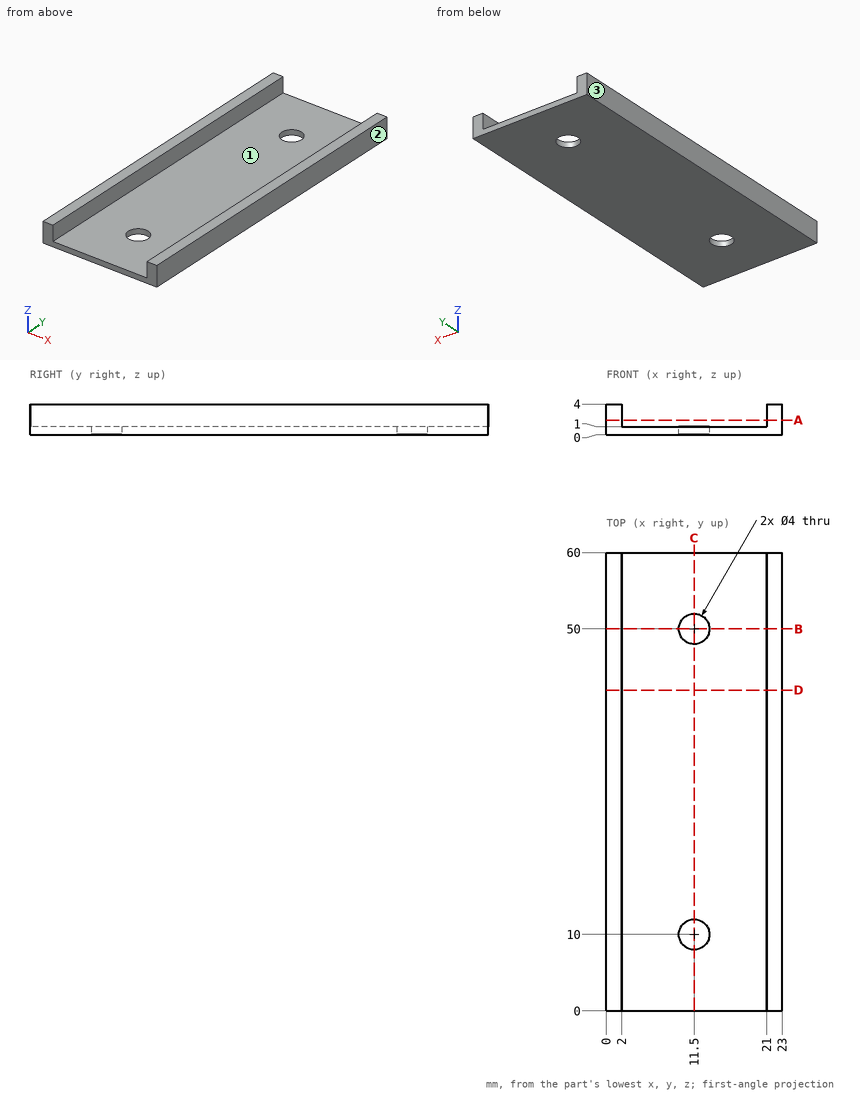
Design review of the part shown in the three views and the two pictorial views. Dimensions are in mm from the part's minimum x, y and z. Give positions to 0.01 mm unless a question says otherwise; leave off trailing zeros. Loops run counter-clockwise (first coordinate to the right, second up) from the corner with the lowest first, then second, coordinate; pieces in that order, holes last. Notation, with made-up numbers: M 9.25,17.5 L 48.25,17.5 A22 cw 48.25,26.5 Z; hole C 40,33.25 d7. An arc over 180 degrees is marked long. Write item = value, one per line.
Q1. We need section B-B (y = 50). Give the boundary of the cut face in (x, z), plus the area to 3 significant figures.
Output values:
outline = M 0,0 L 9.5,0 L 9.5,1 L 2,1 L 2,4 L 0,4 Z; M 13.5,0 L 23,0 L 23,4 L 21,4 L 21,1 L 13.5,1 Z
area = 31.0 mm^2
Q2. Draft analysis for pull direction X (two halves, no side actions). For the marked faces 1, 2 and 3, state which applies: +X half, -X half, draft (parallel to the pull), parting line (faces both ways), or undercut.
Output values:
face_1 = undercut
face_2 = +X half
face_3 = -X half
Q3. We need section C-C (x = 11.5). Give the boundary of the cut face in (y, z), plus the area to 3 significant figures.
Output values:
outline = M 0,0 L 8,0 L 8,1 L 0,1 Z; M 12,0 L 48,0 L 48,1 L 12,1 Z; M 52,0 L 60,0 L 60,1 L 52,1 Z
area = 52.0 mm^2
Q4. To check wall thickness, follow line 1 (Y direction, x = 11.5, z = 0.4); line 2 (X direction, y = 55, z = 2.1); line 3 (Z direction, x = 9.5, y = 4). State the ranges of each line that lie inside material, in increasing order. Write a range as [from, to].
Output values:
line_1 = [0, 8], [12, 48], [52, 60]
line_2 = [0, 2], [21, 23]
line_3 = [0, 1]
Q5. Insertion check: pin 1 (1 mm diameter, centred on x = 17.5, z = 3, fed in from -Y); pin 2 (6 mm diameter, centred on x = 9, y = 45, fed in from +Z). Each pin has a flat end and moves straight along its axis. Give the tip position at first contact, or say it passes through.
Output values:
pin_1 = through
pin_2 = 1
Q6. We need section A-A (z = 1.9). Give the boundary of the cut face in (x, y).
Output values:
outline = M 0,0 L 2,0 L 2,60 L 0,60 Z; M 21,0 L 23,0 L 23,60 L 21,60 Z
Q7. We need section D-D (y = 42). Give the boundary of the cut face in (x, z), plus the area to 3 significant figures.
Output values:
outline = M 0,0 L 23,0 L 23,4 L 21,4 L 21,1 L 2,1 L 2,4 L 0,4 Z
area = 35.0 mm^2
